For this review, take the finished solid that the model builds, in its own axes (mm). Coordinates: 2 decimals unless noted, no trailing zeros. Loops run counter-clockwise (first coordinate to the right, second up) from the corner with the lowest first, then second, coordinate; pieces in that order, holes last. Notation, with made-up numbers: (79, 55) - (123, 55) arc R14 ccw to (123, 71) - close; hole circle Ø6 at (42, 4.25). An arc over 180 degrees is marked (long way). One line per item, written item: value. Start each with the question number.
1. Insertion check: pin 1 (1 mm diameter, centred on x = 0.5, y = 1.5, fed in from -Z). The pin has a flat end and moves straight along its axis. Give the tip position at first contact, or say it passes through.
2. Take a section at D-D, the plane y = -2. State the section outline as (x, z) points, and give its area (3 significant figures).
3. To check wall thickness, follow line 1 (X direction, y = 0, z = 0.2); line 2 (X direction, y = 4.75, z = 0.15); line 3 (X direction, y = -1.25, z = 0.25). State the ranges of each line that lie inside material, in increasing order. Write a range as from..to.
4. Take a section at C-C, the plane x = 0. State the section outline as (y, z) points (3 decimals), and give its area (3 significant figures).
5. Take a section at A-A, the plane y = 3.5. State the section outline as (x, z) points, and give its area (3 significant figures).
6. Take a section at B-B, the plane z = 0.1. State the section outline as (x, y) points (3 decimals), and give its area (3 significant figures).
```python
from build123d import *

# Parameters (mm, degrees)
DODANIE_WYCI_GNI_CIE1_DEPTH = 0.4


with BuildPart() as part:
    # Szkic1 → Dodanie-wyciągnięcie1 (new body)
    with BuildSketch(Plane.XY):
        with BuildLine():
            Line((0.25, -4.975), (0.4, -4.375))
            Line((0.4, -4.375), (0.4, -1.175))
            Line((0.4, -1.175), (0.6, -1.175))
            Line((0.6, -1.175), (1, -0.925))
            Line((1, -0.925), (1, 0.825))
            Line((1, 0.825), (0.813333333, 4.325))
            Line((0.813333333, 4.325), (0.45, 4.975))
            Line((0.45, 4.975), (0.3, 4.575))
            Line((0.3, 4.575), (0.5, 0.825))
            Line((0.5, 0.825), (0.5, -0.075))
            ThreePointArc((0.5, -0.075), (0, -0.575), (-0.5, -0.075))
            Line((-0.5, -0.075), (-0.5, 0.825))
            Line((-0.5, 0.825), (-0.3, 4.575))
            Line((-0.3, 4.575), (-0.45, 4.975))
            Line((-0.45, 4.975), (-0.813333333, 4.325))
            Line((-0.813333333, 4.325), (-1, 0.825))
            Line((-1, 0.825), (-1, -0.925))
            Line((-1, -0.925), (-0.6, -1.175))
            Line((-0.6, -1.175), (-0.4, -1.175))
            Line((-0.4, -1.175), (-0.4, -4.375))
            Line((-0.4, -4.375), (-0.25, -4.975))
            Line((-0.25, -4.975), (0.25, -4.975))
        make_face()
    extrude(amount=DODANIE_WYCI_GNI_CIE1_DEPTH)


solid = part.part
```
Solutions:
1. pin 1: z = 0
2. outline: (-0.4, 0) - (0.4, 0) - (0.4, 0.4) - (-0.4, 0.4) - close
2. area: 0.320 mm2
3. line 1: -1..-0.5, 0.5..1
3. line 2: -0.58..-0.37, 0.37..0.58
3. line 3: -0.4..0.4
4. outline: (-4.975, 0) - (-0.575, 0) - (-0.575, 0.4) - (-4.975, 0.4) - close
4. area: 1.76 mm2
5. outline: (-0.86, 0) - (-0.36, 0) - (-0.36, 0.4) - (-0.86, 0.4) - close; (0.36, 0) - (0.86, 0) - (0.86, 0.4) - (0.36, 0.4) - close
5. area: 0.400 mm2
6. outline: (-1, -0.925) - (-0.6, -1.175) - (-0.4, -1.175) - (-0.4, -4.375) - (-0.25, -4.975) - (0.25, -4.975) - (0.4, -4.375) - (0.4, -1.175) - (0.6, -1.175) - (1, -0.925) - (1, 0.825) - (0.813, 4.325) - (0.45, 4.975) - (0.3, 4.575) - (0.5, 0.825) - (0.5, -0.075) arc R0.5 cw to (-0.5, -0.075) - (-0.5, 0.825) - (-0.3, 4.575) - (-0.45, 4.975) - (-0.813, 4.325) - (-1, 0.825) - close
6. area: 9.43 mm2
